Geometry: final body of the model. Coordinates: model frame, mm. A direction names the side the tool comes from. Coordinates: 2 decimals unless noted, no trailing zeros. Loops run counter-clockwise (first coordinate to the right, second up) from the corner with the lowest first, then second, coordinate; pieces in that order, holes last. Notation, with made-up numbers: (1, -8.5) - (50, -8.5) arc R25 ccw to (50, 14.5) - close; hole circle Ø2 at (44, 78). An arc over 180 degrees is marked (long way). Return JSON: item names as keys, results as strings.
from build123d import *

# Parameters (mm, degrees)
F0_R     = 1.55
F0_R_2   = 14.25
F0_R_3   = 1.75
F0_W     = 12
F0_H     = 2
F1_DEPTH = 3
F2_DEPTH = 7
F3_R     = 2
F3_R_2   = 1.99999


# Not quite as in the source:
# - a fillet or chamfer is up to 0.001 mm smaller than in the source, because OpenCascade refuses the exact size


with BuildPart() as f1:
    # F0 (on Top) → F1 (new body)
    with BuildSketch(Plane.XY):
        Polygon((12.5, -15), (15, -15), (15, 15), (-15, 15), (-15, -15), (-12.5, -15), (-6, -15), (6, -15), align=None)
        with Locations((-12, -12)):
            Circle(F0_R, mode=Mode.SUBTRACT)
        with Locations((12, -12)):
            Circle(F0_R, mode=Mode.SUBTRACT)
        with Locations((-12, 12)):
            Circle(F0_R, mode=Mode.SUBTRACT)
        Circle(F0_R_2, mode=Mode.SUBTRACT)
        with Locations((12, 12)):
            Circle(F0_R, mode=Mode.SUBTRACT)
        Polygon((-6, -17), (-6, -15), (-12.5, -15), (-12.5, -20.8), (-6, -20.8), align=None)
        with Locations((-9.2, -18)):
            Circle(F0_R_3, mode=Mode.SUBTRACT)
        with Locations((0, -16)):
            Rectangle(F0_W, F0_H)
        Polygon((12.5, -20.8), (12.5, -15), (6, -15), (6, -17), (6, -20.8), align=None)
        with Locations((9.2, -18)):
            Circle(F0_R_3, mode=Mode.SUBTRACT)
    extrude(amount=F1_DEPTH)

    # F0 (on Top) → F2 (join)
    with BuildSketch(Plane.XY):
        with Locations((0, -16)):
            Rectangle(F0_W, F0_H)
        Polygon((-6, -17), (-6, -15), (-12.5, -15), (-12.5, -20.8), (-6, -20.8), align=None)
        with Locations((-9.2, -18)):
            Circle(F0_R_3, mode=Mode.SUBTRACT)
        Polygon((12.5, -20.8), (12.5, -15), (6, -15), (6, -17), (6, -20.8), align=None)
        with Locations((9.2, -18)):
            Circle(F0_R_3, mode=Mode.SUBTRACT)
    extrude(amount=F2_DEPTH)

    # F3 (call 1 of 12: OpenCascade refuses the feature's edges together)
    f3_edges = [f1.edges().sort_by_distance(p)[0] for p in [
        (15, -15, 1.5),
    ]]
    fillet(f3_edges, radius=F3_R)

    # F3#2 (call 2 of 12)
    f3_2_edges = [f1.edges().sort_by_distance(p)[0] for p in [
        (-15, -15, 1.5),
    ]]
    fillet(f3_2_edges, radius=F3_R)

    # F3#3 (call 3 of 12)
    f3_3_edges = [f1.edges().sort_by_distance(p)[0] for p in [
        (-15, 15, 1.5),
    ]]
    fillet(f3_3_edges, radius=F3_R)

    # F3#4 (call 4 of 12)
    f3_4_edges = [f1.edges().sort_by_distance(p)[0] for p in [
        (15, 15, 1.5),
    ]]
    fillet(f3_4_edges, radius=F3_R)

    # F3#5 (call 5 of 12)
    f3_5_edges = [f1.edges().sort_by_distance(p)[0] for p in [
        (-12.5, -20.8, 3.5),
    ]]
    fillet(f3_5_edges, radius=F3_R)

    # F3#6 (call 6 of 12)
    f3_6_edges = [f1.edges().sort_by_distance(p)[0] for p in [
        (-6, -20.8, 3.5),
    ]]
    fillet(f3_6_edges, radius=F3_R)

    # F3#7 (call 7 of 12)
    f3_7_edges = [f1.edges().sort_by_distance(p)[0] for p in [
        (6, -20.8, 3.5),
    ]]
    fillet(f3_7_edges, radius=F3_R)

    # F3#8 (call 8 of 12)
    f3_8_edges = [f1.edges().sort_by_distance(p)[0] for p in [
        (12.5, -20.8, 3.5),
    ]]
    fillet(f3_8_edges, radius=F3_R)

    # F3#9 (call 9 of 12)
    f3_9_edges = [f1.edges().sort_by_distance(p)[0] for p in [
        (12.5, -15, 5),
    ]]
    fillet(f3_9_edges, radius=F3_R)

    # F3#10 (call 10 of 12)
    f3_10_edges = [f1.edges().sort_by_distance(p)[0] for p in [
        (-12.5, -15, 5),
    ]]
    fillet(f3_10_edges, radius=F3_R)

    # F3#11 (call 11 of 12) (radius 2 in the source; OpenCascade refuses exactly that, so slightly less here)
    f3_11_edges = [f1.edges().sort_by_distance(p)[0] for p in [
        (0, -17, 7),
    ]]
    fillet(f3_11_edges, radius=F3_R_2)

    # F3#12 (call 12 of 12)
    f3_12_edges = [f1.edges().sort_by_distance(p)[0] for p in [
        (0, -17, 0),
    ]]
    fillet(f3_12_edges, radius=F3_R)


solid = f1.part
Item 1: First-contact query: pin 1 Ø5 at (x, y) = (-10, -2.5) entering from +Z; pin 2 Ø8 at (x, y) = (8, -13.5) entering from -Z; pin 3 Ø4 at (y, z) = (-16.5, 4.5) entering from +X; pin 4 Ø1.1 at (y, z) = (-17, 3) entering from -X. Flat tips, straight axial feed; report the tip coordinate or a pass-through.
Worked out:
{"pin 1": "through", "pin 2": "z = 0", "pin 3": "x = 12.5", "pin 4": "x = -12.5"}
Item 2: Reachability of faces 1 (the face through (-11.9, -15.57, 5.03)), 2 (the face through (0, -15, 5)), 3 (the face through (6.57, -20.2, 3.45)), 4 (the face through (8.972, -16.265, 3.451)) from +Z, -Z, +X, -X, +Y, -Y: full face, straight path, thin tool, end or side. Return the list, or none.
Worked out:
{"face 1": "+Z, -X, +Y", "face 2": "+Z, +X, -X, +Y", "face 3": "+Z, -Z, -Y", "face 4": "+Z, -Z"}
Item 3: Ray query, probe 1 along Y at (x, z) = (9.2, 4); probe 2 along Y at (x, z) = (9.2, 2); probe 3 along Y at (x, z) = (12, 1.05). Return the intervals inside material, ascending. Write a range as from..to.
Worked out:
{"probe 1": "-20.8..-19.75, -16.25..-15", "probe 2": "-20.8..-19.75, -16.25..-10.88, 10.88..15", "probe 3": "-20.12..-13.55, -10.45..-7.69, 7.69..10.45, 13.55..15"}
Item 4: Mould query, pull axis X, two halves, no side actions, for faces 5 (the face through (13.163, -5.458, 1.479)), 6 (the face through (0.08, -16.4, 0.57)), 7 (the face through (-12.5, -17.3, 2.7)), 8 (the face through (0, 15, 1)). Classes: +X half, -X half, draft (parallel to the pull), parting line (faces both ways), or undercut.
Worked out:
{"face 5": "undercut", "face 6": "undercut", "face 7": "-X half", "face 8": "draft"}
Item 5: Section query C-C, the plane y = 0. Return loops of the section in (x, z), and give its area (3 significant figures).
Worked out:
{"outline": "(-15, 0) - (-14.25, 0) - (-14.25, 3) - (-15, 3) - close; (14.25, 0) - (15, 0) - (15, 3) - (14.25, 3) - close", "area": "4.50 mm^2"}
Item 6: Section query B-B, the plane z = 4. Return loops of the section in (x, y).
Worked out:
{"outline": "(-12.5, -18.8) arc R2 ccw to (-10.5, -20.8) - (-8, -20.8) arc R2 ccw to (-6, -18.8) - (-6, -17) - (6, -17) - (6, -18.8) arc R2 ccw to (8, -20.8) - (10.5, -20.8) arc R2 ccw to (12.5, -18.8) - (12.5, -17) arc R2 ccw to (10.5, -15) - (-10.5, -15) arc R2 ccw to (-12.5, -17) - close; hole circle Ø3.5 at (-9.2, -18); hole circle Ø3.5 at (9.2, -18)"}
Item 7: Section query A-A, the plane y = -18. Return loops of the section in (x, z).
Worked out:
{"outline": "(-12.5, 0) - (-10.95, 0) - (-10.95, 7) - (-12.5, 7) - close; (-7.45, 0) - (-6, 0) - (-6, 7) - (-7.45, 7) - close; (6, 0) - (7.45, 0) - (7.45, 7) - (6, 7) - close; (10.95, 0) - (12.5, 0) - (12.5, 7) - (10.95, 7) - close"}
